Could you check a few things on this model? Use its own coordinates, in mm. Face numbers are marked on the shaded views. A direction names the side the tool comes from. Coordinates: 2 decimals unless noted, no trailing zeros. Write each loop counter-clockwise with the first axis right and the second up, starting at its lowest first coordinate (ties: lowest second). Pieces come first, ordered by that corner, then holes.
Item 1: If I drill on probe 1 along Z at (x, y) = (15, 11); probe 2 along X at (y, z) = (2, 31.5); probe 3 along Z at (x, y) = (-8, 9.75), over which ranges is the centre line in solid material (lowest first)?
Item 2: Thinking about a two-plate mould opening in X: for the marked faces 1, 2, 3 and 4, which applies, +X half, -X half, draft (parallel to the pull), parting line (faces both ways), or undercut?
Item 3: Which directions (+Z, -Z, +X, -X, +Y, -Y) give clear straight access to the entire face, cutting with the end or side of a thin tool? Please do the marked faces 5, 6, 7 and 8.
Item 4: For P1, Ø3, axis at y = 2, z = 9, coming from the -X side; P2, Ø1.8, axis at x = 5.5, z = 30, coming from the +Y side; P3, Ø2.5, axis at x = -12, y = 8, coming from the +Z side, each with a flat end and sliding along its axis, tell me the tip position at first contact or that it passes through.
Item 5: I want a section at D-D on x = -8. Please give me the cut outline in (y, z), then the cut area to 3 significant figures.
Item 6: I want a section at A-A on x = 16.5. Please give me the cut outline in (y, z), then the cut area to 3 significant figures.
Item 7: I want a section at B-B on z = 29. Please give me the cut outline in (x, y).
Item 8: I want a section at C-C on x = -3. Please give me the cut outline in (y, z), then the cut area to 3 significant figures.
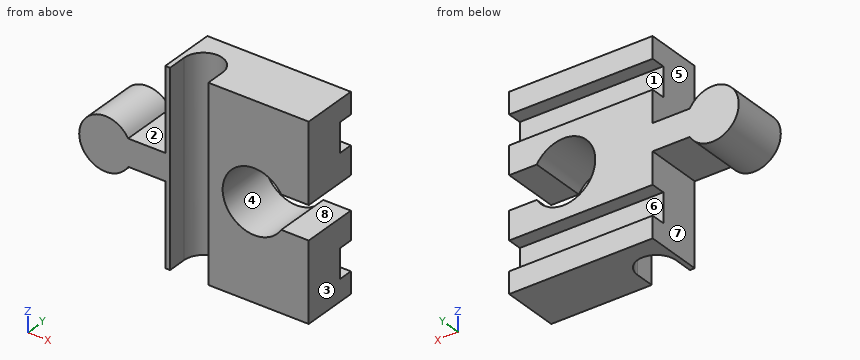
Autodesk Inventor part; units mm, degrees
ref_plane "YZ Plane" through (0, 0, 0) normal (1, 0, 0) x (0, 1, 0)
ref_plane "XZ Plane" through (0, 0, 0) normal (0, 1, 0) x (-1, 0, 0)
ref_plane "XY Plane" through (0, 0, 0) normal (0, 0, 1) x (1, 0, 0)
sketch "Sketch1" plane through (0, 0, 0) normal (0, 1, 0) x (-1, 0, 0)
  line L0 (9.5606, 37.6724) -> (-20.4394, 37.6724)
  line L1 (-20.4394, -2.3276) -> (9.5606, -2.3276)
  line L2 (17.3267, 20.4724) -> (9.5606, 20.4724)
  line L3 (9.5606, 14.8724) -> (17.3267, 14.8724)
  arc A0 (17.3267, 14.8724) -> (17.3267, 20.4724) centre (22.0606, 17.6724) ccw
  line L4 (9.5606, -2.3276) -> (9.5606, 14.8724)
  line L5 (9.5606, 20.4724) -> (9.5606, 37.6724)
  arc A1 (-14.6894, 14.1724) -> (-14.6894, 21.1724) centre (-9.0644, 17.6724) ccw
  line L6 (-14.6894, 21.1724) -> (-20.4394, 21.1724)
  line L7 (-14.6894, 14.1724) -> (-20.4394, 14.1724)
  line L8 (-20.4394, 37.6724) -> (-20.4394, 21.1724)
  line L9 (-20.4394, 14.1724) -> (-20.4394, -2.3276)
  point P0 (0, 0)
  dimension "d0" = 30
  dimension "d1" = 40
  dimension "d2" = 17.2
  dimension "d5" = 17.2
  dimension "d10" = 12.5
  dimension "d12" = 7.7661
  dimension "d17" = 13.25
  dimension "d18" = 20
  dimension "d19" = 16.5
  dimension "d20" = 16.5
extrude "Extrusion1" add sketch "Sketch1" along normal blind 11.9
sketch "Sketch2" plane through (0, 11.9, 0) normal (0, 1, 0) x (1, 0, 0)
  line L0 (-9.5606, -20.4724) -> (-9.5606, -37.6724)
  line L1 (-9.5606, -33.1724) -> (20.4769, -33.1724)
  line L2 (20.4769, -33.1724) -> (20.4769, -27.0724)
  line L3 (20.4769, -27.0724) -> (-9.5606, -27.0724)
  line L4 (-9.5606, -27.0724) -> (-9.5606, -33.1724)
  line L5 (-9.5606, -37.6724) -> (20.4394, -37.6724)
  line L6 (-9.5606, -8.2724) -> (20.4769, -8.2724)
  line L7 (20.4769, -8.2724) -> (20.4769, -2.1724)
  line L8 (20.4769, -2.1724) -> (-9.5606, -2.1724)
  line L9 (-9.5606, -2.1724) -> (-9.5606, -8.2724)
  line L10 (20.4394, 2.3276) -> (-9.5606, 2.3276)
  line L11 (-9.5606, 2.3276) -> (-9.5606, -14.8724)
  point P0 (0, 0)
  dimension "d24" = 6.1
  dimension "d25" = 4.5
  dimension "d26" = 6.1
  dimension "d27" = 4.5
  dimension "d35" = 0
extrude "Extrusion2" cut sketch "Sketch2" against normal blind 3
sketch "Sketch3" plane through (20.4394, 0, -2.3276) normal (0, 0, -1) x (-1, 0, 0)
  line L0 (21, 0) -> (29, 0)
  line L1 (29, 0) -> (29, 4)
  line L2 (21, 4) -> (21, 0)
  arc A0 (29, 4) -> (21, 4) centre (25, 4) ccw
  line L3 (30, 0) -> (30, 11.9)
  point P0 (20.4394, 0)
  dimension "d34" = 9
extrude "Extrusion3" cut sketch "Sketch3" against normal through all
properties part number "traintrack"
Response values:
1. probe 1: z = -2.33 to 2.17, 8.27 to 14.17, 21.17 to 27.07, 33.17 to 37.67
1. probe 2: x = -9.56 to -8.56, -0.56 to 20.44
1. probe 3: z = -2.33 to 2.17, 8.27 to 27.07, 33.17 to 37.67
2. face 1: draft
2. face 2: undercut
2. face 3: +X half
2. face 4: undercut
3. face 5: +Z, +Y, -Y
3. face 6: +X, -X, +Y
3. face 7: -Z, +Y, -Y
3. face 8: +X, +Y, -Y
4. P1: stops at x = -9.56
4. P2: stops at y = 8.9
4. P3: stops at z = 20.47
5. outline: (6.04, -2.33) - (11.9, -2.33) - (11.9, 2.17) - (8.9, 2.17) - (8.9, 8.27) - (11.9, 8.27) - (11.9, 27.07) - (8.9, 27.07) - (8.9, 33.17) - (11.9, 33.17) - (11.9, 37.67) - (6.04, 37.67) - close
5. area: 198 mm2
6. outline: (0, -2.33) - (11.9, -2.33) - (11.9, 2.17) - (8.9, 2.17) - (8.9, 8.27) - (11.9, 8.27) - (11.9, 14.17) - (0, 14.17) - close; (0, 21.17) - (11.9, 21.17) - (11.9, 27.07) - (8.9, 27.07) - (8.9, 33.17) - (11.9, 33.17) - (11.9, 37.67) - (0, 37.67) - close
6. area: 356 mm2
7. outline: (-9.56, 0) - (-8.56, 0) - (-8.56, 4) arc R4 cw to (-0.56, 4) - (-0.56, 0) - (20.44, 0) - (20.44, 8.9) - (-9.56, 8.9) - close
8. outline: (7.68, -2.33) - (11.9, -2.33) - (11.9, 2.17) - (8.9, 2.17) - (8.9, 8.27) - (11.9, 8.27) - (11.9, 27.07) - (8.9, 27.07) - (8.9, 33.17) - (11.9, 33.17) - (11.9, 37.67) - (7.68, 37.67) - close
8. area: 132 mm2
